```python
from build123d import *

# Parameters (mm, degrees)
F1_DEPTH = 63.5
F2_DEPTH = 25.4
F3_DEPTH = 7.9375
F0_W     = 25.4
F0_H     = 19.0499985942
F4_DEPTH = 25.4
F6_R     = 6.35


with BuildPart() as f1:
    # F0 (on Front) → F1 (new body, symmetric)
    with BuildSketch(Plane.XZ):
        Polygon((-41.275, 9.525), (-41.275, -9.525), (41.275, -9.525), (41.275, 9.525), (22.2250014058, 9.525), align=None)
    extrude(amount=F1_DEPTH, both=True)

    # F0 (on Front) → F2 (join, symmetric)
    with BuildSketch(Plane.XZ):
        with BuildLine():
            Line((22.2250014058, 9.525), (41.275, 9.525))
            Line((41.275, 9.525), (41.275, 25.4321699366))
            ThreePointArc((41.275, 25.4321699366), (46.2876837818, 37.0091173484), (58.1601289922, 41.275))
            Line((58.1601289922, 41.275), (60.325, 41.275))
            Line((60.325, 41.275), (60.325, 60.3249985942))
            Line((60.325, 60.3249985942), (58.6486777751, 60.3249985942))
            ThreePointArc((58.6486777751, 60.3249985942), (55.7661237808, 60.3297402447), (52.8929969389, 60.0967549152))
            ThreePointArc((52.8929969389, 60.0967549152), (30.9924833678, 48.5739038915), (22.2250014058, 25.4321699366))
            Line((22.2250014058, 25.4321699366), (22.2250014058, 9.525))
        make_face()
    extrude(amount=F2_DEPTH, both=True)

    # F0 (on Front) → F3 (join, symmetric)
    with BuildSketch(Plane.XZ):
        with BuildLine():
            add(Edge.make_bspline(
                [(-41.275, 9.525), (-40.9022124169, 41.6161306688), (0.6165533939, 57.971909164), (52.8929969389, 60.0967549152)],
                knots=[0, 0, 0, 0, 108.2857694169, 108.2857694169, 108.2857694169, 108.2857694169], degree=3))
            Line((-41.275, 9.525), (22.2250014058, 9.525))
            Line((22.2250014058, 9.525), (22.2250014058, 25.4321699366))
            ThreePointArc((22.2250014058, 25.4321699366), (30.9924833678, 48.5739038915), (52.8929969389, 60.0967549152))
        make_face()
    extrude(amount=F3_DEPTH, both=True)

    # F0 (on Front) → F4 (join, symmetric)
    with BuildSketch(Plane.XZ):
        with Locations((73.025, 50.7999992971)):
            Rectangle(F0_W, F0_H)
    extrude(amount=F4_DEPTH, both=True)

    # F0 (on Front) → F5 (revolve)
    with BuildSketch(Plane.XZ):
        Polygon((85.725, 66.675), (85.725, 60.3249985942), (85.725, 41.275), (85.725, 38.1), (111.125, 38.1), (111.125, 66.675), align=None)
    revolve(axis=Axis((85.725, 0, 52.3875), (0, 0, 1)))

    # F6
    f6_edges = [f1.edges().sort_by_distance(p)[0] for p in [
        (-41.275, -63.5, 0),
        (41.275, -63.5, 0),
        (41.275, 63.5, 0),
        (-41.275, 63.5, 0),
    ]]
    fillet(f6_edges, radius=F6_R)


solid = f1.part
```
Here's how the part is built. I have some questions about the finished solid (model axes, mm). A direction names the side the tool comes from. Coordinates: 2 decimals unless noted, no trailing zeros. Loops run counter-clockwise (first coordinate to the right, second up) from the corner with the lowest first, then second, coordinate; pieces in that order, holes last. Notation, with made-up numbers: (-24, 11.25) - (35, 11.25) arc R12 ccw to (35, 23.25) - close; hole circle Ø11 at (40, -10). An arc over 180 degrees is marked (long way). Return JSON: item names as keys, results as strings. Group by question number.
Item 1: If we section it at A-A on z = 1: Write out the boundary of the cut face in (x, y) (3 decimals).
Item 2: If we section it at C-C on x = 81.5: Write out the boundary of the cut face in (y, z) (3 decimals).
Item 3: If we section it at B-B on y = 23: Write out the boundary of the cut face in (x, z) (3 decimals).
Item 4: I need wall thicknesses on line 1 (Z direction, x = -2, y = -18.5) (3 decimals); line 2 (Y direction, x = -1, z = 29); line 3 (Y direction, x = 42, z = 46). Which ranges of each line are inside material? Lowest first, please. Write a range as from..to.
Item 5: On a 3-axis mill with a long thin cutter (end or side, diameter ignored), from which of +Z, -Z, +X, -X, +Y, -Y can I reach the whole of each face in a straight line? I mean faces 1 (the face through (22.225, -17, 18)), 2 (the face through (86, 0, 38.1)), 3 (the face through (22.225, 17, 18)). Say none if no direction works.
Item 6: If we section it at D-D on y = -21.5: Write out the boundary of the cut face in (x, z) (3 decimals).
Item 7: Will these pins go through, and if not, where does the flat tip stop? P1, Ø15, axis at x = 47.5, z = 41, coming from the -Y side; P2, Ø6, axis at x = -7.5, y = 24.5, coming from the +Z side (3 decimals); P3, Ø15, axis at x = -10, z = 30.5, coming from the -Y side.
Calculated:
{
 "1": {"outline": "(-41.275, -57.15) arc R6.35 ccw to (-34.925, -63.5) - (34.925, -63.5) arc R6.35 ccw to (41.275, -57.15) - (41.275, 57.15) arc R6.35 ccw to (34.925, 63.5) - (-34.925, 63.5) arc R6.35 ccw to (-41.275, 57.15) - close"},
 "2": {"outline": "(-25.4, 41.275) - (-25.046, 41.275) - (-25.046, 38.1) - (25.046, 38.1) - (25.046, 41.275) - (25.4, 41.275) - (25.4, 60.325) - (25.046, 60.325) - (25.046, 66.675) - (-25.046, 66.675) - (-25.046, 60.325) - (-25.4, 60.325) - close"},
 "3": {"outline": "(-41.275, -9.525) - (41.275, -9.525) - (41.275, 25.432) arc R15.875 cw to (58.16, 41.275) - (74.947, 41.275) - (74.947, 38.1) - (96.503, 38.1) - (96.503, 66.675) - (74.947, 66.675) - (74.947, 60.325) - (58.649, 60.325) arc R34.925 ccw to (22.225, 25.432) - (22.225, 9.525) - (-41.275, 9.525) - close"},
 "4": {"line 1": "z = -9.525..9.525", "line 2": "y = -7.94..7.94", "line 3": "y = -25.4..25.4"},
 "5": {"face 1": "+Z, -X, -Y", "face 2": "-Z, +X, +Y, -Y", "face 3": "+Z, -X, +Y"},
 "6": {"outline": "(-41.275, -9.525) - (41.275, -9.525) - (41.275, 25.432) arc R15.875 cw to (58.16, 41.275) - (72.201, 41.275) - (72.201, 38.1) - (99.249, 38.1) - (99.249, 66.675) - (72.201, 66.675) - (72.201, 60.325) - (58.649, 60.325) arc R34.925 ccw to (22.225, 25.432) - (22.225, 9.525) - (-41.275, 9.525) - close"},
 "7": {"P1": "stops at y = -25.4", "P2": "stops at z = 9.525", "P3": "stops at y = -7.94"}
}
